The model under review builds one solid part; all positions refer to its coordinate system, in mm. Face numbers are marked on the shaded views. Coordinates: 2 decimals unless noted, no trailing zeros. Write each loop counter-clockwise with the first axis right and the second up, starting at its lowest first coordinate (ties: lowest second). Pieces come first, ordered by that corner, then holes.
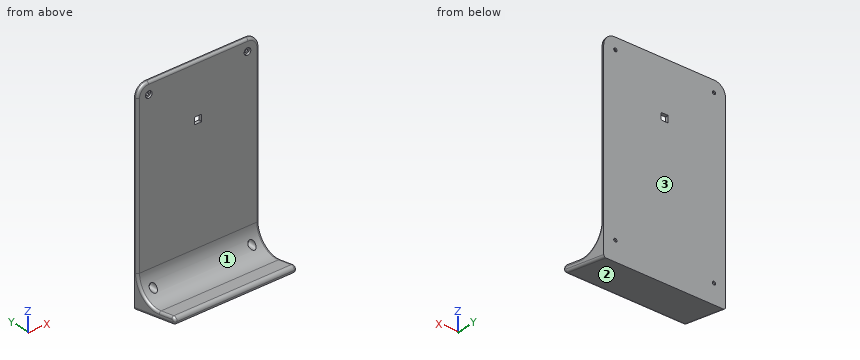
```python
from build123d import *

# Parameters (mm, degrees)
BOSS_EXTRUDE1_DEPTH = 1.5
SKETCH3_W           = 54.19363593
SKETCH3_H           = 15
BOSS_EXTRUDE2_DEPTH = 20
CUT_EXTRUDE2_DEPTH  = 107.861890415
CUT_EXTRUDE4_DEPTH  = 107.861890415
FILLET1_R           = 1.5
SKETCH7_R           = 0.75
CUT_EXTRUDE5_DEPTH  = 109.286974912
SKETCH9_R           = 1.5
CUT_EXTRUDE6_DEPTH  = 5.9
FILLET2_R           = 1
CUT_EXTRUDE7_DEPTH  = 110.092020548


with BuildPart() as part:
    # Sketch1 → Boss-Extrude1 (new body)
    with BuildSketch(Plane(origin=(0, 0, 0), x_dir=(1, 0, 0), z_dir=(0, 1, 0))):
        with BuildLine():
            Line((9.274778516, 0), (53.468414446, 0))
            ThreePointArc((53.468414446, 0), (57.003948352, 1.464466094), (58.468414446, 5))
            Line((58.468414446, 5), (58.468414446, 89.9028))
            Line((58.468414446, 89.9028), (4.274778516, 89.9028))
            Line((4.274778516, 89.9028), (4.274778516, 5))
            ThreePointArc((4.274778516, 5), (5.73924461, 1.464466094), (9.274778516, 0))
        make_face()
    extrude(amount=BOSS_EXTRUDE1_DEPTH)

    # Sketch3 → Boss-Extrude2 (add)
    with BuildSketch(Plane.XZ):
        with Locations((31.371596481, -82.4028)):
            Rectangle(SKETCH3_W, SKETCH3_H)
    extrude(amount=BOSS_EXTRUDE2_DEPTH)

    # Sketch2 → Cut-Extrude2 (cut, through all)
    with BuildSketch(Plane(origin=(58.468414446, 0, 0), x_dir=(0, 0, -1), z_dir=(1, 0, 0))):
        Polygon((89.9028, 1.5), (86.111769915, -20), (89.9028, -20), align=None)
    extrude(amount=-CUT_EXTRUDE2_DEPTH, mode=Mode.SUBTRACT)

    # Sketch4 → Cut-Extrude4 (cut, through all)
    with BuildSketch(Plane.ZY.offset(-4.274778516)):
        with BuildLine():
            Line((-74.9028, 0), (-74.9028, -20))
            Line((-74.9028, -20), (-83.065490079, -20))
            Line((-83.065490079, -20), (-84.562216259, -11.511644029))
            ThreePointArc((-84.562216259, -11.511644029), (-82.416492014, -3.503692127), (-74.9028, 0))
        make_face()
    extrude(amount=-CUT_EXTRUDE4_DEPTH, mode=Mode.SUBTRACT)

    # Fillet1
    fillet1_edges = [part.edges().sort_by_distance(p)[0] for p in [
        (31.371596481, -20, -86.111769915),
        (31.371596481, -20, -83.065490079),
    ]]
    fillet(fillet1_edges, radius=FILLET1_R - 0.0001)  # a hair under: the kernel refuses the full size

    # Sketch7 → Cut-Extrude5 (cut, through all)
    with BuildSketch(Plane(origin=(0, -5, 0), x_dir=(-1, 0, 0), z_dir=(0, -1, 0))):
        with Locations(Location((-53.302878516, 5.0861, 0), (0, 0, 90))):
            Circle(SKETCH7_R)
        with Locations(Location((-9.386278516, 5.0861, 0), (0, 0, 90))):
            Circle(SKETCH7_R)
        with Locations(Location((-9.386278516, 81.1845, 0), (0, 0, 90))):
            Circle(SKETCH7_R)
        with Locations(Location((-53.302878516, 81.1845, 0), (0, 0, 90))):
            Circle(SKETCH7_R)
    extrude(amount=-CUT_EXTRUDE5_DEPTH, mode=Mode.SUBTRACT)

    # Sketch9 → Cut-Extrude6 (cut)
    with BuildSketch(Plane(origin=(0, -5, 0), x_dir=(-1, 0, 0), z_dir=(0, -1, 0))):
        with Locations(Location((-53.302878516, 5.0861, 0), (0, 0, 90))):
            Circle(SKETCH9_R)
        with Locations(Location((-9.386278516, 5.0861, 0), (0, 0, 90))):
            Circle(SKETCH9_R)
        with Locations(Location((-9.386278516, 81.1845, 0), (0, 0, 90))):
            Circle(SKETCH9_R)
        with Locations(Location((-53.302878516, 81.1845, 0), (0, 0, 90))):
            Circle(SKETCH9_R)
    extrude(amount=-CUT_EXTRUDE6_DEPTH, mode=Mode.SUBTRACT)

    # Fillet2
    fillet2_edges = [part.edges().sort_by_distance(p)[0] for p in [
        (4.274778516, 0, -39.9514),
        (4.274778516, -8.630277451, -88.116558763),
        (58.468414446, -8.630277451, -88.116558763),
        (58.468414446, -3.503692127, -82.416492014),
        (58.468414446, -14.875644564, -83.969052201),
        (4.274778516, -3.503692127, -82.416492014),
        (4.274778516, -14.875644564, -83.969052201),
        (58.468414446, -19.464217136, -83.704011232),
        (58.468414446, -19.64909006, -85.817321514),
        (4.274778516, -19.464217136, -83.704011232),
        (4.274778516, -19.64909006, -85.817321514),
        (57.003948352, 0, -1.464466094),
        (31.371596481, 0, 0),
        (5.73924461, 0, -1.464466094),
        (58.468414446, 0, -39.9514),
    ]]
    fillet(fillet2_edges, radius=FILLET2_R)

    # Sketch10 → Cut-Extrude7 (cut, through all)
    with BuildSketch(Plane.XZ):
        with BuildLine():
            Line((32.669578516, -22.1128), (30.019578516, -22.1128))
            ThreePointArc((30.019578516, -22.1128), (29.87815716, -22.171378644), (29.819578516, -22.3128))
            Line((29.819578516, -22.3128), (29.819578516, -24.9628))
            ThreePointArc((29.819578516, -24.9628), (29.87815716, -25.104221356), (30.019578516, -25.1628))
            Line((30.019578516, -25.1628), (32.669578516, -25.1628))
            ThreePointArc((32.669578516, -25.1628), (32.810999872, -25.104221356), (32.869578516, -24.9628))
            Line((32.869578516, -24.9628), (32.869578516, -22.3128))
            ThreePointArc((32.869578516, -22.3128), (32.810999872, -22.171378644), (32.669578516, -22.1128))
        make_face()
    extrude(amount=-CUT_EXTRUDE7_DEPTH, mode=Mode.SUBTRACT)


solid = part.part
```
Item 1: For pin 1 (4 mm diameter, centred on x = 50.5, y = -15.5, fed in from -Z); pin 2 (1.5 mm diameter, centred on x = 52.5, y = -6, fed in from +Z); pin 3 (2.5 mm diameter, centred on x = 9, z = -5.5, fed in from -Y); pin 4 (1.6 mm diameter, centred on y = 0.5, z = -23, fed in from +X), all flat-tipped, find the tip position at first contact; note any pin that passes through.
Solved:
pin 1: stops at z = -87.26
pin 2: stops at z = -83.59
pin 3: stops at y = 0
pin 4: stops at x = 58.47
Item 2: Take a section at C-C, the plane z = -42. Write out the cut boundary in (x, y).
Solved:
outline: (4.27, 1) arc R1 ccw to (5.27, 0) - (57.47, 0) arc R1 ccw to (58.47, 1) - (58.47, 1.5) - (4.27, 1.5) - close
Item 3: Mouldability with a two-part tool opening along Y and no side actions: class the marked faces 1, 2 and 3 as pulls with the +Y half, pulls with the -Y half, needs draft (parallel to the pull), parting line crosses it, or undercut.
Solved:
face 1: undercut
face 2: pulls with the -Y half
face 3: pulls with the +Y half
Item 4: To check wall thickness, follow line 1 along Y through (x, z) = (29, -50.5); line 2 along Z through (x, y) = (45, -6.25); line 3 along Z through (x, y) = (54.5, -2). State the ranges of each line that lie inside material, in increasing order.
Solved:
line 1: y = 0 to 1.5
line 2: z = -88.54 to -84.04
line 3: z = -89.29 to -82.09
